Input: part model. Units: mm. Frame: model coordinates. Face numbers are marked on the shaded views. A direction names the side the tool comes from. Round coordinates to 2 decimals unless told otherwise and drop trailing zeros. Loops run counter-clockwise (first coordinate to the right, second up) from the corner with the lowest first, then second, coordinate; pieces in that order, holes last.
1) Access query for the marked faces 1 and 2. Directions: +Z, -Z, +X, -X, +Y, -Y. A direction counts if a zero-diameter tool reaches every point of the face in a straight line with its end or side. Return the directions, or none.
2) Section C-C, the plane z = 42.8. Return loops of the section in (x, y).
3) Ray query, line 1 along X through (y, z) = (18.8, 50.7); line 2 along X through (y, z) = (-1.15, 42.8); line 3 along Y through (x, z) = (18.8, 49.85). Return the intervals inside material, ascending.
4) Section D-D, the plane x = 15. Return loops of the section in (y, z), and give its area (3 significant figures).
5) Section B-B, the plane y = 15.5. Return loops of the section in (x, z).
6) First-contact query: pin 1 (4 mm diameter, centred on x = 18.8, y = 34.3, fed in from -Z); pin 2 (11.5 mm diameter, centred on x = 27, z = 34, fed in from +Y); pin 3 (2.5 mm diameter, centred on x = 34.3, y = 18.8, fed in from +Z); pin 4 (2 mm diameter, centred on y = 21.5, z = 50, fed in from -X). Flat tips, straight axial feed; report the tip coordinate or a pass-through.
7) Section A-A, the plane x = 18.8. Return loops of the section in (y, z), and give its area (3 significant figures).
Autodesk Inventor part; units mm, degrees
ref_plane "YZ Plane" through (0, 0, 0) normal (1, 0, 0) x (0, 1, 0)
ref_plane "XZ Plane" through (0, 0, 0) normal (0, 1, 0) x (-1, 0, 0)
ref_plane "XY Plane" through (0, 0, 0) normal (0, 0, 1) x (1, 0, 0)
sketch "Sketch1" plane through (0, 0, 0) normal (1, 0, 0) x (0, 1, 0)
  line L0 (0, 0) -> (0, 49.2)
  line L1 (0, 49.2) -> (37.6, 49.2)
  line L2 (37.6, 51.2) -> (-2, 51.2)
  line L3 (-2, 51.2) -> (-2, 0)
  line L4 (37.6, 51.2) -> (37.6, 49.2)
  line L5 (0, 0) -> (-2, 0)
  dimension "d0" = 49.2
  dimension "d1" = 37.6
  dimension "d2" = 2
extrude "Extrusion1" add sketch "Sketch1" along normal blind 37.6
fillet "Fillet1" radius 2 1 edges at (18.8, -2, 51.2)
fillet "Fillet2" radius 2 2 edges at (37.6, -1, 0) (0, -1, 0)
sketch "Sketch2" plane through (0, 37.6, 51.2) normal (0, 0, 1) x (1, 0, 0)
  line L0 (0, -39.6) -> (37.6, -39.6)
  line L1 (0, -39.6) -> (0, -18.8)
  line L2 (0, -37.6) -> (0, 0)
  circle A0 centre (18.794722, -18.794721) radius 15.5
  circle A1 centre (3.294722, -18.794721) radius 1.65
  circle A2 centre (34.3, -18.8) radius 1.65
  circle A3 centre (18.8, -3.3) radius 1.65
  circle A4 centre (18.794722, -18.794721) radius 18.805278
  line L3 (37.6, -37.6) -> (37.6, 0)
  line L4 (37.6, -18.8) -> (37.6, 0)
  line L5 (0, 0) -> (37.6, 0)
  line L6 (37.6, 0) -> (0, 0)
  line L7 (0, 0) -> (0, -18.16472)
  arc A5 (37.6, -18.8) -> (0, -18.8) centre (18.8, -18.8) ccw
  line L8 (18.8, -18.8) -> (18.8, -11.8)
  line L9 (18.8, -11.8) -> (18.8, -25.8)
  line L10 (18.8, -18.8) -> (25.4, -18.8)
  line L11 (25.4, -18.8) -> (12.2, -18.8)
  line L12 (18.8, -11.8) -> (12.2, -11.8)
  line L13 (12.2, -11.8) -> (12.2, -25.8)
  line L14 (12.2, -25.8) -> (25.4, -25.8)
  line L15 (25.4, -25.8) -> (25.4, -11.8)
  line L16 (25.4, -11.8) -> (18.8, -11.8)
  arc A6 (25.4, -11.8) -> (12.2, -11.8) centre (18.8, -14.132381) ccw
  arc A7 (12.2, -25.8) -> (25.4, -25.8) centre (18.8, -23.467619) ccw
  dimension "d8" = 31
  dimension "d7" = 20.8
  dimension "d9" = 3.3
  dimension "d10" = 3.3
  dimension "d11" = 3.3
  dimension "d16" = 7
  dimension "d17" = 14
  dimension "d18" = 6.6
  dimension "d19" = 13.2
  dimension "d20" = 7
  dimension "d21" = 7
extrude "Extrusion2" cut sketch "Sketch2" against normal through all contours A0 A2 | A0 A2 | A3 A0 | A0 A3 | A1 A0 | A0 A1
sketch "Sketch2 outline for Extrusion3" plane through (0, 37.6, 51.2) normal (0, 0, 1) x (1, 0, 0)
  line L0 (0, 0) -> (0, -18.8)
  arc A0 (18.8, 0) -> (0, -18.8) centre (18.8, -18.8) ccw
  line L1 (18.8, 0) -> (0, 0)
  arc A1 (37.6, -18.8) -> (18.8, 0) centre (18.8, -18.8) ccw
  line L2 (37.6, 0) -> (18.8, 0)
  line L3 (37.6, -18.8) -> (37.6, 0)
extrude "Extrusion3" cut sketch "Sketch2 outline for Extrusion3" against normal through all
extrude "Extrusion4" cut sketch "Sketch2" against normal blind 37.6 contours L11 L13 L12 L8 | L10 L15 L14 L9 | L8 L16 L15 L10 | L9 L14 L13 L11 | L12 A6 L16 | L14 A7
sketch "Sketch4" plane through (0, 0, 49.2) normal (0, 1, 0) x (1, 0, 0)
  line L0 (37.6, -2) -> (0, -2)
  line L1 (0, -2) -> (0, 6.4)
  line L2 (0, 47.2) -> (0, 0)
  line L3 (18.8, -2) -> (3.2, -2)
  line L4 (3.2, -2) -> (34.4, -2)
  line L5 (3.2, -2) -> (3.2, 6.4)
  circle A0 centre (3.2, 6.4) radius 1.6
  line L6 (34.4, -2) -> (34.4, 6.4)
  circle A1 centre (34.4, 6.4) radius 1.6
  point P0 (0, 49.2)
  dimension "d24" = 8.4
  dimension "d25" = 15.6
  dimension "d26" = 31.2
  dimension "d27" = 3.2
  dimension "d28" = 3.2
extrude "Extrusion5" cut sketch "Sketch4" against normal blind 37.6
properties part number "motor mount"
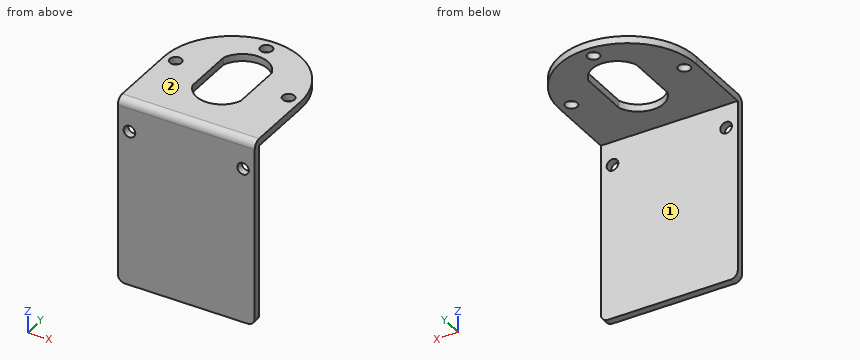
Final values:
1. face 1: -Z, +X, -X, +Y
1. face 2: +Z, +X, -X, +Y, -Y
2. outline: (0, -2) - (1.6, -2) - (1.6, 0) - (0, 0) - close; (4.8, -2) - (32.8, -2) - (32.8, 0) - (4.8, 0) - close; (36, -2) - (37.6, -2) - (37.6, 0) - (36, 0) - close
3. line 1: x = 0 to 1.64, 4.94 to 12.2, 25.4 to 32.65, 35.95 to 37.6
3. line 2: x = 0 to 1.6, 4.8 to 32.8, 36 to 37.6
3. line 3: y = -1.89 to 7.13, 30.47 to 32.65, 35.95 to 37.6
4. outline: (-2, 0) - (0, 0) - (0, 49.2) - (8.25, 49.2) - (8.25, 51.2) - (0, 51.2) arc R2 ccw to (-2, 49.2) - close; (29.35, 49.2) - (37.21, 49.2) - (37.21, 51.2) - (29.35, 51.2) - close
4. area: 134 mm2
5. outline: (0, 49.2) - (12.2, 49.2) - (12.2, 51.2) - (0, 51.2) - close; (25.4, 49.2) - (37.6, 49.2) - (37.6, 51.2) - (25.4, 51.2) - close
6. pin 1: stops at z = 49.2
6. pin 2: stops at y = 0
6. pin 3: passes through
6. pin 4: stops at x = 0.08
7. outline: (-2, 0) - (0, 0) - (0, 49.2) - (7.13, 49.2) - (7.13, 51.2) - (0, 51.2) arc R2 ccw to (-2, 49.2) - close; (30.47, 49.2) - (32.65, 49.2) - (32.65, 51.2) - (30.47, 51.2) - close; (35.95, 49.2) - (37.6, 49.2) - (37.6, 51.2) - (35.95, 51.2) - close
7. area: 123 mm2
